```python
from build123d import *

# Parameters (mm, degrees)
F1_DEPTH    = 19.05
F2_T1_DEPTH = 171.45
F3_W        = 12.7
F3_H        = 38.1
F7_R        = 3.175
F8_R        = 3.175


# Not quite as in the source:
# - a fillet or chamfer that OpenCascade refuses, or shapes differently, is made with other operations: its cross-section is extruded or revolved along the edge and cut away or added


with BuildPart() as f1:
    # F0 (on Front) → F1 (new body, symmetric)
    with BuildSketch(Plane.XZ):
        Polygon((-38.1, 57.15), (-26.9875, 0), (26.9875, 0), (38.1, 57.15), (38.1, 101.6), (-38.1, 101.6), align=None)
    extrude(amount=F1_DEPTH, both=True)

    # F2: fillet of radius 19.05 on 2 edges, made by hand

    # F2_s2 → F2_t1 (cut)
    with BuildSketch(Plane.YZ.offset(-85.725)):
        with BuildLine():
            ThreePointArc((0, 101.6), (-13.4703841816, 96.0203841816), (-19.05, 82.55))
            Line((-19.05, 82.55), (-19.05, 101.6))
            Line((-19.05, 101.6), (0, 101.6))
        make_face()
        with BuildLine():
            ThreePointArc((0, 101.6), (13.4703841816, 96.0203841816), (19.05, 82.55))
            Line((19.05, 82.55), (19.05, 101.6))
            Line((19.05, 101.6), (0, 101.6))
        make_face()
    extrude(amount=F2_T1_DEPTH, mode=Mode.SUBTRACT)

    # F3 (on Front) → F4 (revolve)
    with BuildSketch(Plane.XZ):
        with Locations((6.35, 101.6)):
            Rectangle(F3_W, F3_H)
    revolve(axis=Axis((0, 0, 41.275), (0, 0, -1)))

    # F5 (on Right) → F6 (revolve)
    with BuildSketch(Plane.YZ):
        with BuildLine():
            Line((-5.08, 158.115), (-5.08, 102.235))
            add(Edge.make_bspline(
                [(-5.08, 102.235), (17.145, 102.235), (17.145, 130.175), (17.145, 158.115), (-5.08, 158.115)],
                knots=[3.1415926536, 3.1415926536, 3.1415926536, 4.7123889804, 4.7123889804, 6.2831853072, 6.2831853072, 6.2831853072], degree=2, weights=[1, 0.7071067812, 1, 0.7071067812, 1]))
        make_face()
    revolve(axis=Axis((0, -5.08, 55.275326029), (0, 0, -1)))

    # F7
    f7_edges = [f1.edges().sort_by_distance(p)[0] for p in [
        (-38.1, 0, 57.15),
        (38.1, 0, 57.15),
    ]]
    fillet(f7_edges, radius=F7_R)

    # F8
    f8_edges = [f1.edges().sort_by_distance(p)[0] for p in [
        (32.514564, -19.05, 28.424903),
        (-32.514564, -19.05, 28.424903),
        (-32.514564, 19.05, 28.424903),
        (-38.1, 19.05, 70.002908),
        (-38.085374, 19.05, 57.151409),
        (38.1, 19.05, 70.002908),
        (38.085374, 19.05, 57.151409),
        (32.514564, 19.05, 28.424903),
        (-38.085374, -19.05, 57.151409),
        (-38.1, -19.05, 70.002908),
        (38.1, -19.05, 70.002908),
        (38.085374, -19.05, 57.151409),
        (-38.1, -13.470384, 96.020384),
        (-38.1, 13.470384, 96.020384),
        (38.1, 13.470384, 96.020384),
        (38.1, -13.470384, 96.020384),
    ]]
    fillet(f8_edges, radius=F8_R)


solid = f1.part
```
Here's how the part is built. I have some questions about the finished solid (model axes, mm). A direction names the side the tool comes from. Give positions to 0.01 mm unless a question says otherwise; leave off trailing zeros. Write each question's results on one line, items separated by ' | '.
Item 1: For pin 1 Ø1 at (x, z) = (15.5, 120.5) entering from -Y; pin 2 Ø10 at (y, z) = (-8.5, 40.5) entering from -X; pin 3 Ø1 at (x, z) = (-14.5, 80) entering from -Y, each with a flat end and sliding along its axis, tell me the tip position at first contact or that it passes through.
Output:
pin 1: stops at y = -19.6 | pin 2: stops at x = -35.83 | pin 3: stops at y = -19.05
Item 2: If I drill on L1, parallel to Y at x = 7, z = 71; L2, parallel to Z at x = -8.5, y = 10.5, over which ranges is the centre line in solid material (lowest first)?
Output:
L1: y = -19.05 to 19.05 | L2: z = 0 to 98.45, 113.36 to 146.99
Item 3: On a 3-axis mill with a long thin cutter (end or side, diameter ignored), from which of +Z, -Z, +X, -X, +Y, -Y can I reach the whole of each face in a straight line? I mean faces 1 (the face through (0, -19.05, 42)), 2 (the face through (32.437, -0.222, 28.027)). Say none if no direction works.
Output:
face 1: -Z, +X, -X, -Y | face 2: -Z, +X, +Y, -Y
Item 4: We'd pull the mould along Z, two halves only. Please class faces 3 (the face through (-2.75, 12.4, 105.2)), 4 (the face through (-32.59, -0.22, 28.82)), 5 (the face through (37.15, -18.14, 70.18)): pulls with the +Z half, pulls with the -Z half, needs draft (parallel to the pull), parting line crosses it, or undercut.
Output:
face 3: undercut | face 4: pulls with the -Z half | face 5: needs draft
